Autodesk Inventor part; units mm, degrees
sketch "Sketch1" plane through (0, 0, 0) normal (0, 1, 0) x (-1, 0, 0)
  point P0 (0, 0)
sketch "Sketch2" plane through (0, 0, 0) normal (0, 1, 0) x (-1, 0, 0)
  line L0 (0, 0) -> (-65, 0)
  line L1 (-65, 0) -> (-65, -46)
  line L2 (-65, -46) -> (0, -46)
  line L3 (0, -46) -> (0, 0)
  dimension "d0" = 65
  dimension "d1" = 46
extrude "Extrusion1" add sketch "Sketch2" along normal blind 3
sketch "Sketch3" plane through (0, 3, 0) normal (0, 1, 0) x (1, 0, 0)
  circle A0 centre (32.5, 37) radius 3.1
  line L0 (65, 46) -> (0, 46)
  line L1 (65, 0) -> (65, 46)
  line L2 (12.5, 40.1) -> (52.5, 40.1)
  line L3 (0, 46) -> (0, 0)
  line L4 (12.5, 33.9) -> (52.5, 33.9)
  arc A1 (12.5, 40.1) -> (12.5, 33.9) centre (12.5, 37) ccw
  arc A2 (52.5, 33.9) -> (52.5, 40.1) centre (52.5, 37) ccw
  point P0 (63.5, 46)
  point P1 (1.5, 46)
  point P2 (32.5, 46)
  point P3 (32.5, 46)
  point P4 (32.5, 46)
  point P5 (32.5, 40.1)
  point P6 (32.5, 40.1)
  point P7 (32.5, 33.9)
  dimension "d5" = 6.2
  dimension "d6" = 0
  dimension "d7" = 9
  dimension "d18" = 40
  dimension "d19" = 0
extrude "Extrusion2" cut sketch "Sketch3" against normal blind 1.2
sketch "Sketch6" plane through (0, 3, 0) normal (0, 1, 0) x (1, 0, 0)
  line L0 (0, 0) -> (65, 0)
  line L1 (65, 0) -> (65, 46)
  line L2 (0, 0) -> (65, 0)
  line L3 (65, 0) -> (65, 46)
  line L4 (65, 46) -> (0, 46)
  line L5 (0, 46) -> (0, 0)
  line L6 (1.2, 44.8) -> (63.8, 44.8)
  line L7 (63.8, 44.8) -> (63.8, 1.2)
  line L8 (63.8, 1.2) -> (1.2, 1.2)
  line L9 (1.2, 1.2) -> (1.2, 44.8)
  dimension "d13" = 1.2
extrude "Extrusion4" add sketch "Sketch6" along normal blind 3
fillet "Fillet2" radius 1.5 4 edges at (0, 3, 0) (65, 3, 0) (65, 3, -46) (0, 3, -46)
equation "\"d0\" = length + thickness"
equation "\"d1\" = width + thickness"
equation "\"d2\" = thickness"
equation "\"d5\" = mag_diameter"
equation "\"d8\" = mag_thickness"
equation "\"d13\" = 0.4 * thickness"
equation "\"d14\" = thickness"
equation "\"d16\" = 0.5 * thickness"
equation "\"length\" = 62"
equation "\"width\" = 43"
equation "\"thickness\" = 3"
equation "\"mag_thickness\" = 1.2"
equation "\"mag_diameter\" = 6.2"
properties part number "mag_case_v3"
Design review of the part built by this model. Coordinates are the model's own, in mm. A direction names the side the tool comes from. Coordinates: 2 decimals unless noted, no trailing zeros. Loops run counter-clockwise (first coordinate to the right, second up) from the corner with the lowest first, then second, coordinate; pieces in that order, holes last.
Q1. Tool access review of faces 1 (the face through (0, 3, -23)), 2 (the face through (9.4, 2.4, -37.1)): name each direction out of +Z, -Z, +X, -X, +Y, -Y from which nothing blocks a thin tool from reaching the whole face with its end or side.
Reported:
face 1: +Z, -Z, -X, +Y, -Y
face 2: +Y
Q2. We need section C-C on x = 35. State the section outline as (y, z) points, and give its area (3 significant figures).
Reported:
outline: (0, -46) - (6, -46) - (6, -44.8) - (3, -44.8) - (3, -40.1) - (1.8, -40.1) - (1.8, -33.9) - (3, -33.9) - (3, -1.2) - (6, -1.2) - (6, 0) - (0, 0) - close
area: 138 mm2
Q3. We need section B-B on z = -6. State the section outline as (x, y) points.
Reported:
outline: (0, 0) - (65, 0) - (65, 6) - (63.8, 6) - (63.8, 3) - (1.2, 3) - (1.2, 6) - (0, 6) - close
Q4. We need section D-D on z = -37. State the section outline as (x, y) points, and give its area (3 significant figures).
Reported:
outline: (0, 0) - (65, 0) - (65, 6) - (63.8, 6) - (63.8, 3) - (55.6, 3) - (55.6, 1.8) - (9.4, 1.8) - (9.4, 3) - (1.2, 3) - (1.2, 6) - (0, 6) - close
area: 147 mm2
Q5. The part is to be moulded in two halves that separate along X. For faces 3 (the face through (32, 2, -40.1)), 4 (the face through (1, 6, -23)), 5 (the face through (64.55, 2.96, -45.57)), say which applies: +X half, -X half, draft (parallel to the pull), parting line (faces both ways), or undercut.
Reported:
face 3: undercut
face 4: draft
face 5: +X half
Q6. To check wall thickness, follow line 1 (X direction, y = 4.75, z = -15.5); line 2 (Z direction, x = 4.5, y = 4.9); line 3 (Y direction, x = 21.5, z = -33.5). State the ranges of each line that lie inside material, in increasing order.
Reported:
line 1: x = 0 to 1.2, 63.8 to 65
line 2: z = -46 to -44.8, -1.2 to 0
line 3: y = 0 to 3
Q7. We need section A-A on y = 4.95. State the section outline as (x, z) points.
Reported:
outline: (0, -44.5) arc R1.5 ccw to (1.5, -46) - (63.5, -46) arc R1.5 ccw to (65, -44.5) - (65, -1.5) arc R1.5 ccw to (63.5, 0) - (1.5, 0) arc R1.5 ccw to (0, -1.5) - close; hole (1.2, -44.8) - (63.8, -44.8) - (63.8, -1.2) - (1.2, -1.2) - close
Q8. For pin 1 (1.5 mm diameter, centred on x = 38, z = -27.5, fed in from +Y); pin 2 (3 mm diameter, centred on x = 22, z = -38.5, fed in from +Y), all flat-tipped, find the tip position at first contact; note any pin that passes through.
Reported:
pin 1: stops at y = 3
pin 2: stops at y = 1.8
